The listing builds one solid part. Answer for the finished solid, in the listing's coordinates (mm). A direction names the side the tool comes from. Round coordinates to 2 decimals unless told otherwise and drop trailing zeros. Write each loop counter-clockwise with the first axis right and the second up, starting at its lowest first coordinate (ties: lowest second). Pieces come first, ordered by that corner, then holes. Notation, with made-up numbers: (80.5, 36) - (124.5, 36) arc R23 ccw to (124.5, 70) - close; hole circle Ø6 at (74, 71). An arc over 180 degrees is marked (long way). Return JSON: item names as keys, results as strings. Group by question number.
from build123d import *

# Parameters (mm, degrees)
EXTRUDE_1621_DEPTH     = 1.6
SKETCH3_W              = 18.561492042
SKETCH3_H              = 6.1
SKETCH3_W_2            = 18.663069739
CUT_EXTRUDE_3212_DEPTH = 135.908052021
CUT_EXTRUDE_3564_DEPTH = 1.6


with BuildPart() as part:
    # Sketch1 → Extrude 1621 (new body)
    with BuildSketch(Plane(origin=(0, 0, 0), x_dir=(0, 0, -1), z_dir=(1, 0, 0))):
        Polygon((0, -1.6), (0, 0), (2.25, 0), (2.25, 12.5), (-132.25, 12.5), (-132.25, 0), (-128, 0), (-128, -1.6), (-120, -1.6), (-120, 0), (-98, 0), (-98, -1.6), (-82.5, -1.6), (-82.5, 0), (-45.5, 0), (-45.5, -1.6), (-30, -1.6), (-30, 0), (-8, 0), (-8, -1.6), align=None)
    extrude(amount=EXTRUDE_1621_DEPTH)

    # Mirror1: part across plane


with BuildPart() as part_1:
    add(part.part)
    add(part.part.mirror(Plane(origin=(1.6, 12.5, 0), x_dir=(0, 0, 1), z_dir=(0, 1, 0))))

    # Sketch3 → Cut-Extrude 3212 (cut, through all)
    with BuildSketch(Plane(origin=(0, 0, 0), x_dir=(0, 0, -1), z_dir=(1, 0, 0))):
        with Locations((-109.620995127, 1.45)):
            Rectangle(SKETCH3_W, SKETCH3_H)
        with Locations((-23.26706902, 1.45)):
            Rectangle(SKETCH3_W_2, SKETCH3_H)
        with BuildLine():
            ThreePointArc((-70, 0), (-73.5, 3.5), (-77, 0))
            Line((-77, 0), (-70, 0))
        make_face()
        with BuildLine():
            ThreePointArc((-55, 0), (-58.5, 3.5), (-62, 0))
            Line((-62, 0), (-55, 0))
        make_face()
    extrude(amount=CUT_EXTRUDE_3212_DEPTH, mode=Mode.SUBTRACT)

    # Sketch4 → Cut-Extrude 3564 (cut)
    with BuildSketch(Plane(origin=(0, 0, 0), x_dir=(0, 0, -1), z_dir=(1, 0, 0))):
        with BuildLine():
            Line((-11.375951178, 21.428362829), (-4.243604313, 12.928362829))
            ThreePointArc((-4.243604313, 12.928362829), (-4.613374813, 8.701866671), (-8.839870972, 9.071637171))
            Line((-8.839870972, 9.071637171), (-15.972217837, 17.571637171))
            ThreePointArc((-15.972217837, 17.571637171), (-15.602447336, 21.798133329), (-11.375951178, 21.428362829))
        make_face()
        with BuildLine():
            Line((-121.131197482, 21.428362829), (-113.998850617, 12.928362829))
            ThreePointArc((-113.998850617, 12.928362829), (-114.368621117, 8.701866671), (-118.595117275, 9.071637171))
            Line((-118.595117275, 9.071637171), (-125.72746414, 17.571637171))
            ThreePointArc((-125.72746414, 17.571637171), (-125.35769364, 21.798133329), (-121.131197482, 21.428362829))
        make_face()
        with BuildLine():
            Line((-23.875951178, 21.428362829), (-16.743604313, 12.928362829))
            ThreePointArc((-16.743604313, 12.928362829), (-17.113374813, 8.701866671), (-21.339870972, 9.071637171))
            Line((-21.339870972, 9.071637171), (-28.472217837, 17.571637171))
            ThreePointArc((-28.472217837, 17.571637171), (-28.102447336, 21.798133329), (-23.875951178, 21.428362829))
        make_face()
        with BuildLine():
            Line((-108.631197482, 21.428362829), (-101.498850617, 12.928362829))
            ThreePointArc((-101.498850617, 12.928362829), (-101.868621117, 8.701866671), (-106.095117275, 9.071637171))
            Line((-106.095117275, 9.071637171), (-113.22746414, 17.571637171))
            ThreePointArc((-113.22746414, 17.571637171), (-112.85769364, 21.798133329), (-108.631197482, 21.428362829))
        make_face()
        with BuildLine():
            Line((-96.131197482, 21.428362829), (-88.998850617, 12.928362829))
            ThreePointArc((-88.998850617, 12.928362829), (-89.368621117, 8.701866671), (-93.595117275, 9.071637171))
            Line((-93.595117275, 9.071637171), (-100.72746414, 17.571637171))
            ThreePointArc((-100.72746414, 17.571637171), (-100.35769364, 21.798133329), (-96.131197482, 21.428362829))
        make_face()
    extrude(amount=CUT_EXTRUDE_3564_DEPTH, mode=Mode.SUBTRACT)


solid = part_1.part
(1) Find section C-C (z = 58.5). Write down the section's boundary in (x, y).
(2) Find section A-A (y = 11). Write down the section's boundary in (x, z).
(3) For faces 4 (the cylindrical face through (0.8, 3.5, 73.4)), 5 (the flat face through (0.79, 13.26, 109.61)), determine the directions among +Z, -Z, +X, -X, +Y, -Y from which every point of the face is accessible in a straight line to the end or side of a thin tool.
(4) Consider line 1 (Z direction, x = 0.5, y = 4.25); line 2 (Z direction, x = 1.05, y = 8.25); line 3 (Z direction, x = 0.8, y = 18.25). Determine where each line is inside the solid, lowest interval first.
(5) Determine the mould class of faces 1 (the flat face through (0, 12, 66)), 2 (the cylindrical face through (0.8, 3.5, 58.4)), 3 (the cylindrical face through (0.789, 8.745, 4.563)) for opening direction Y: +Y half, -Y half, draft (parallel to the pull), parting line (faces both ways), or undercut.
(6) Find section B-B (z = 25). Write down the section's boundary in (x, y), plus the area to 3 significant figures.
(7) Flat-ended cylindrical pins translate along their axes: pin 1 (0.5 mm diameter, centred on x = 0.5, z = 51, fed in from -Y); pin 2 (0.5 mm diameter, centred on x = 0.5, y = -1, fed in from +Z); pin 3 (0.5 mm diameter, centred on x = 0.5, z = 22.5, fed in from -Y). Find the tip coordinate at first contact, or state that the pin passes through.
Check sheet entries:
{
 "1": {"outline": "(0, 3.5) - (1.6, 3.5) - (1.6, 25) - (0, 25) - close"},
 "2": {"outline": "(0, -2.25) - (1.6, -2.25) - (1.6, 3.54) - (0, 3.54) - close; (0, 10.46) - (1.6, 10.46) - (1.6, 16.04) - (0, 16.04) - close; (0, 22.96) - (1.6, 22.96) - (1.6, 88.3) - (0, 88.3) - close; (0, 95.21) - (1.6, 95.21) - (1.6, 100.8) - (0, 100.8) - close; (0, 107.71) - (1.6, 107.71) - (1.6, 113.3) - (0, 113.3) - close; (0, 120.21) - (1.6, 120.21) - (1.6, 132.25) - (0, 132.25) - close"},
 "3": {"face 4": "+X, -X, -Y", "face 5": "+X, -X"},
 "4": {"line 1": "z = -2.25 to 13.94, 32.6 to 100.34, 118.9 to 132.25", "line 2": "z = -2.25 to 5.34, 7.74 to 17.84, 20.24 to 90.1, 92.5 to 102.6, 105 to 115.1, 117.5 to 132.25", "line 3": "z = -2.25 to 8.71, 16.4 to 21.21, 28.9 to 93.46, 101.16 to 105.96, 113.66 to 118.46, 126.16 to 132.25"},
 "5": {"face 1": "draft", "face 2": "-Y half", "face 3": "undercut"},
 "6": {"outline": "(0, 4.5) - (1.6, 4.5) - (1.6, 13.43) - (0, 13.43) - close; (0, 22.26) - (1.6, 22.26) - (1.6, 25) - (0, 25) - close", "area": "18.7 mm^2"},
 "7": {"pin 1": "stops at y = 0", "pin 2": "stops at z = 128", "pin 3": "stops at y = 4.5"}
}
